Input: part model. Units: mm. Frame: model coordinates. A direction names the side the tool comes from. Coordinates: 2 decimals unless noted, no trailing zeros. Loops run counter-clockwise (first coordinate to the right, second up) from the corner with the lowest first, then second, coordinate; pieces in that order, holes last.
(1) Section C-C, the plane x = 10.5. Return loops of the section in (y, z).
(2) Set-up query: faces 1 (the face through (21, 2, -1)), 2 (the face through (10.9, 0, 3)), 3 (the face through (9, -1, 4.5)), 4 (the face through (16, -1, 0.5)). Return all of +Z, -Z, +X, -X, +Y, -Y with unobstructed straight access to the full face (end or side cutting, diameter ignored); none if empty.
(3) Contact query for flat-ended pins moving along their axis: P1, Ø1.5, axis at y = -2, z = 3, coming from the +X side; P2, Ø1.2, axis at y = -1.5, z = 2.5, coming from the -X side; P3, Ø2, axis at y = 1.5, z = -1.5, coming from the +X side; P4, Ø0.8, axis at x = 10, y = -1, coming from the -Z side. Output: stop coordinate, or through.
(4) Section D-D, the plane z = 2.5. Return loops of the section in (x, y), then the cut area to 3 significant figures.
(5) Mould query, pull axis X, two halves, no side actions, for faces 5 (the face through (14.1, 0, 3)), 6 (the face through (12.522, 0.833, 3.398)), 7 (the face through (7.9, -3, 2)), 8 (the face through (2, 2, 0)). Classes: released by +X, released by -X, zero draft, split by the parting line, or undercut.
(6) Section B-B, the plane x = 5.5. Return loops of the section in (y, z).
(7) Section A-A, the plane y = 2. Return loops of the section in (x, z), then the cut area to 3 significant figures.
(8) Line query: L1, parallel to Z at x = 9.9, y = -1.5; L2, parallel to Y at x = 10, z = -2.5; L3, parallel to Y at x = 16.5, z = 2.5. Output: solid intervals per line, ascending.
```python
from build123d import *

# Parameters (mm, degrees)
BOSS_EXTRUDE1_DEPTH      = 4
BOSS_EXTRUDE2_START      = 4
SKETCH2_R                = 1
BOSS_EXTRUDE2_DEPTH      = 17
BOSS_EXTRUDE3_DEPTH      = 4.6
BOSS_EXTRUDE3_DEPTH_BACK = 4.6
BOSS_EXTRUDE3_START      = 12.5
SKETCH3_R                = 1
CUT_EXTRUDE1_REACH       = 29.604
SKETCH4_W                = 3.2
SKETCH4_H                = 3.5
CUT_EXTRUDE2_DEPTH       = 3.2


with BuildPart() as part:
    # Sketch1 → Boss-Extrude1 (new body)
    with BuildSketch(Plane(origin=(0, 0, 0), x_dir=(1, 0, 0), z_dir=(0, 1, 0))):
        Polygon((0, 0), (4.551348998, -6.5), (20.448651002, -6.5), (25, 0), align=None)
    extrude(amount=BOSS_EXTRUDE1_DEPTH)

    # Sketch2 → Boss-Extrude2 (add)
    with BuildSketch(Plane(origin=(0, 0, 0), x_dir=(0, 0, -1), z_dir=(1, 0, 0)).offset(BOSS_EXTRUDE2_START)):
        with BuildLine():
            Line((0, 0), (2.5, 0))
            ThreePointArc((2.5, 0), (4.5, 2), (2.5, 4))
            Line((2.5, 4), (0, 4))
            Line((0, 4), (0, 0))
        make_face()
        with Locations((2.5, 2)):
            Circle(SKETCH2_R, mode=Mode.SUBTRACT)
    extrude(amount=BOSS_EXTRUDE2_DEPTH)

    # Sketch3 → Boss-Extrude3 (add, two sides: drawn at the far end of the back side and taken through both)
    with BuildSketch(Plane(origin=(0, 0, 0), x_dir=(0, 0, -1), z_dir=(1, 0, 0)).offset(BOSS_EXTRUDE3_START - BOSS_EXTRUDE3_DEPTH_BACK)):
        with BuildLine():
            Line((-4.5, 0), (-0.5, 0))
            Line((-0.5, 0), (-0.5, -1.5))
            ThreePointArc((-0.5, -1.5), (-2.5, -3.5), (-4.5, -1.5))
            Line((-4.5, -1.5), (-4.5, 0))
        make_face()
        with Locations((-2.5, -1.5)):
            Circle(SKETCH3_R, mode=Mode.SUBTRACT)
    extrude(amount=BOSS_EXTRUDE3_DEPTH + BOSS_EXTRUDE3_DEPTH_BACK)

    # Sketch4 → Cut-Extrude1 (cut, up to next)
    with BuildSketch(Plane.XY.offset(6.5), mode=Mode.PRIVATE) as cut_extrude1_sk1:
        with Locations((12.5, -1.75)):
            Rectangle(SKETCH4_W, SKETCH4_H)
    cut_extrude1_tool1 = extrude(cut_extrude1_sk1.sketch, amount=-CUT_EXTRUDE1_REACH, mode=Mode.PRIVATE) & part.part
    add(cut_extrude1_tool1.solids().sort_by_distance((12.5, -1.75, 6.5))[0], mode=Mode.SUBTRACT)

    # Sketch5 → Cut-Extrude2 (cut)
    with BuildSketch(Plane.ZY.offset(-14.1)):
        with BuildLine():
            Line((1.983840692, 0.94613564), (-2.5, 0))
            Line((-2.5, 0), (0.5, 0))
            ThreePointArc((0.5, 0), (3.84408243, -3.607947443), (1.983840692, 0.94613564))
        make_face()
    extrude(amount=CUT_EXTRUDE2_DEPTH, mode=Mode.SUBTRACT)


solid = part.part
```
Report:
1. outline: (-1.5, 0.5) - (0, 0.5) - (0, -2.5) arc R2 ccw to (4, -2.5) - (4, 6.5) - (0, 6.5) - (0, 4.5) - (-1.5, 4.5) arc R2 ccw to start; hole circle Ø2 at (-1.5, 2.5); hole circle Ø2 at (2, -2.5)
2. face 1: -Z, +X, +Y, -Y
2. face 2: -Y
2. face 3: +Z, +X, -X, -Y
2. face 4: -Z, +X, -X, -Y
3. P1: stops at x = 17.1
3. P2: passes through
3. P3: stops at x = 21
3. P4: stops at z = 0.5
4. outline: (1.75, 0) - (7.9, 0) - (7.9, -0.5) - (10.9, -0.5) - (10.9, 1) - (14.1, 1) - (14.1, -0.5) - (17.1, -0.5) - (17.1, 0) - (23.25, 0) - (23.25, 4) - (1.75, 4) - close; (7.9, -3.5) - (10.9, -3.5) - (10.9, -2.5) - (7.9, -2.5) - close; (14.1, -3.5) - (17.1, -3.5) - (17.1, -2.5) - (14.1, -2.5) - close
4. area: 91.8 mm2
5. face 5: undercut
5. face 6: undercut
5. face 7: released by -X
5. face 8: zero draft
6. outline: (0, -2.5) arc R2 ccw to (4, -2.5) - (4, 6.5) - (0, 6.5) - close; hole circle Ø2 at (2, -2.5)
7. outline: (0, 0) - (4, 0) - (4, -1.5) - (21, -1.5) - (21, 0) - (25, 0) - (20.45, 6.5) - (4.55, 6.5) - close; (4, -4.5) - (21, -4.5) - (21, -3.5) - (4, -3.5) - close
7. area: 175 mm2
8. L1: z = 0.5 to 1.5, 3.5 to 4.5
8. L2: y = 0 to 1, 3 to 4
8. L3: y = -3.5 to -2.5, -0.5 to 4
